The listing builds one solid part. Answer for the finished solid, in the listing's coordinates (mm). Give positions to 0.01 mm unless a question says otherwise; leave off trailing zeros. Loops run counter-clockwise (first coordinate to the right, second up) from the corner with the lowest first, then second, coordinate; pieces in that order, holes last. Notation, with made-up numbers: M -28.75,35.25 L -16.75,35.25 A17 ccw -16.75,65.25 Z; hole C 28,-21.75 d4. An arc over 180 degrees is marked long. Return JSON: item names as keys, results as strings.
from build123d import *

# Parameters (mm, degrees)
SKETCH1_R           = 45
SKETCH1_R_2         = 2.175
SKETCH1_R_3         = 3.975
SKETCH1_R_4         = 2.5
BOSS_EXTRUDE1_DEPTH = 5


with BuildPart() as part:
    # Sketch1 → Boss-Extrude1 (new body)
    with BuildSketch(Plane.XY):
        Circle(SKETCH1_R)
        with Locations((12, 0)):
            Circle(SKETCH1_R_2, mode=Mode.SUBTRACT)
        with Locations((0, 12)):
            Circle(SKETCH1_R_2, mode=Mode.SUBTRACT)
        with Locations((-12, 0)):
            Circle(SKETCH1_R_2, mode=Mode.SUBTRACT)
        with Locations((0, -12)):
            Circle(SKETCH1_R_2, mode=Mode.SUBTRACT)
        Circle(SKETCH1_R_3, mode=Mode.SUBTRACT)
        with Locations((-26.516504294, 26.516504294)):
            Circle(SKETCH1_R_4, mode=Mode.SUBTRACT)
        with Locations((26.516504294, -26.516504294)):
            Circle(SKETCH1_R_4, mode=Mode.SUBTRACT)
    extrude(amount=BOSS_EXTRUDE1_DEPTH)


solid = part.part
(1) The part is cut by section A-A (x = 0). Determine the outline of the cut face in (y, z) (3 decimals).
Values follow:
{"outline": "M -45,0 L -14.175,0 L -14.175,5 L -45,5 Z; M -9.825,0 L -3.975,0 L -3.975,5 L -9.825,5 Z; M 3.975,0 L 9.825,0 L 9.825,5 L 3.975,5 Z; M 14.175,0 L 45,0 L 45,5 L 14.175,5 Z"}
(2) The part is cut by section C-C (x = 12). Determine the outline of the cut face in (y, z) (1 decimal).
Values follow:
{"outline": "M -43.4,0 L -2.2,0 L -2.2,5 L -43.4,5 Z; M 2.2,0 L 43.4,0 L 43.4,5 L 2.2,5 Z"}
(3) Straight lines are drawn through the part: line 1 along Y through (x, z) = (0, 2.2) (3 decimals); line 2 along X through (y, z) = (1.5, 0.7) (3 decimals); line 3 along Y through (x, z) = (-12, 3.65) (1 decimal). For each, find the intervals that lie inside material, in ascending order.
Values follow:
{"line 1": "-45 to -14.175, -9.825 to -3.975, 3.975 to 9.825, 14.175 to 45", "line 2": "-44.975 to -13.575, -10.425 to -3.681, 3.681 to 10.425, 13.575 to 44.975", "line 3": "-43.4 to -2.2, 2.2 to 43.4"}
(4) Determine the mould class of faces 1 (the flat face through (9, 1, 0)), 2 (the cylindrical face through (20.765, -39.923, 2.465)), 3 (the cylindrical face through (-24.207, 25.559, 2.465)) for opening direction X: released by +X, released by -X, zero draft, split by the parting line, or undercut.
Values follow:
{"face 1": "zero draft", "face 2": "split by the parting line", "face 3": "undercut"}
(5) The part is cut by section B-B (z = 1.4). Give the number of separate pieces and of enclosed holes in the cut face, and give its area (3 significant figures).
Values follow:
{"separate pieces": "1", "enclosed holes": "7", "area": "6,210 mm²"}
(6) Given pin 1 (4 mm diameter, centred on x = 8.5, y = -34, fed in from -Z); pin 2 (3 mm diameter, centred on x = -8.5, z = 1, fed in from -Y); pin 3 (1.5 mm diameter, centred on x = -6, z = 1, fed in from +Y), each flat-ended and moving along its own axis, determine where each tip first touches the part or whether it passes through.
Values follow:
{"pin 1": "z = 0", "pin 2": "y = -44.45", "pin 3": "y = 44.69"}
